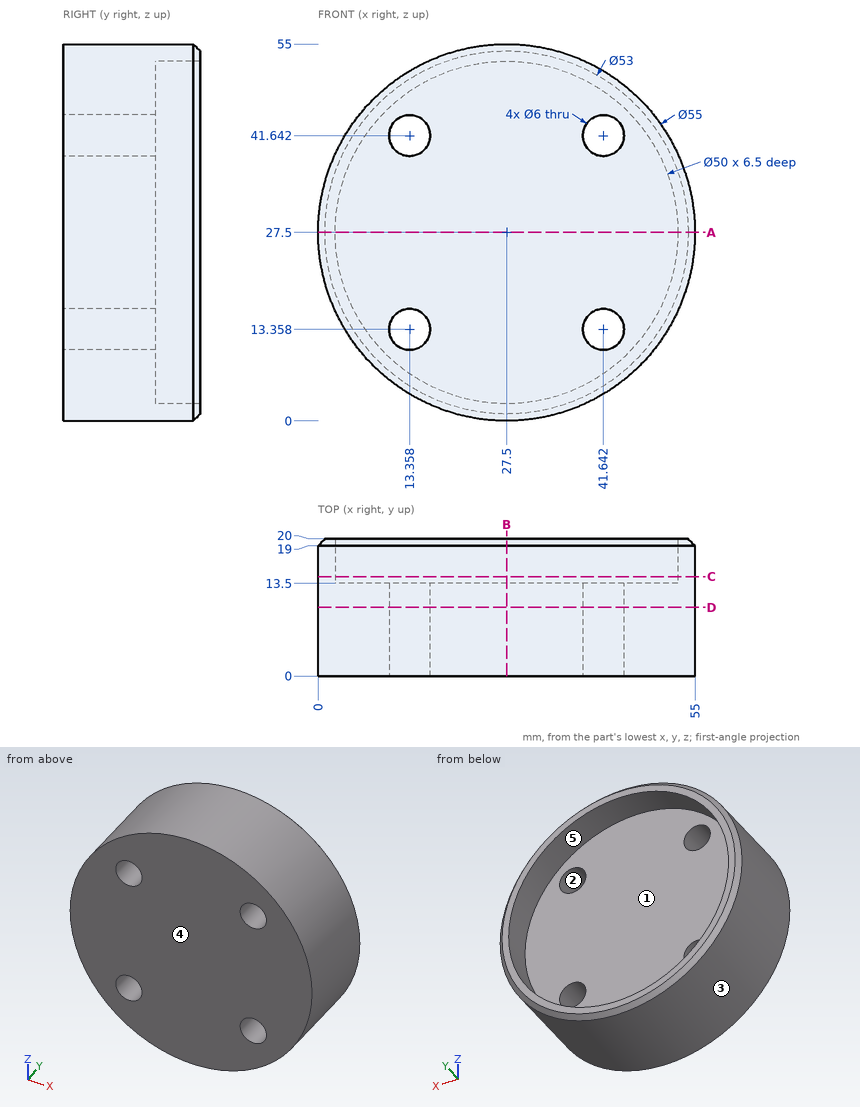
Geometry: see drawing. Coordinates: mm, zero at the bounding-box minimum. A direction names the side the tool comes from. Give positions to 0.01 mm unless a question says otherwise; leave off trailing zeros. Order: outer loops, then holes, each group sorted by start corner. A loop starts at its lowest first (then second) coordinate and runs counter-clockwise, first axis right, second up. Notation, with made-up numbers: (66.5, -32) -> (112.5, -32) arc R19 cw to (112.5, 3) -> close; hole circle Ø11 at (4, 29.25). An arc over 180 degrees is marked (long way). Write each question's results on one line, items separated by ' | '. Start each with the question number.
1) Line query: line 1 (X direction, y = 12, z = 44); line 2 (X direction, y = 11.5, z = 43) (1 decimal); line 3 (Z direction, x = 27.5, y = 16.25). Output: solid intervals per line, ascending. Write a range as from..to.
2) Section D-D (y = 10). Return loops of the section in (x, z), then the cut area to 3 significant figures.
3) Section B-B (x = 27.5). Return loops of the section in (y, z).
4) Section C-C (y = 14.5). Return loops of the section in (x, z), then the cut area to 3 significant figures.
5) Set-up query: the marked faces 1 and 2. Return all of +Z, -Z, +X, -X, +Y, -Y with unobstructed straight access to the full face (end or side cutting, diameter ignored); none if empty.
6) Section A-A (z = 27.5). Return loops of the section in (x, y), then the cut area to 3 significant figures.
7) Draft query along X for the marked faces 3, 4 and 5. Return one class per face: pulls with the +X half, pulls with the -X half, needs draft (parallel to the pull), parting line crosses it, or undercut.
8) First-contact query: pin 1 (2 mm diameter, centred on x = 16.5, z = 42.5, fed in from +Y); pin 2 (8 mm diameter, centred on x = 26, y = 2, fed in from -Z); pin 3 (2 mm diameter, centred on x = 18, y = 4.5, fed in from -Z); pin 4 (3.5 mm diameter, centred on x = 13.36, z = 13.36, fed in from +Y). Flat tips, straight axial feed; report the tip coordinate or a pass-through.
Calculated:
1) line 1: 5.5..11.5, 15.21..39.79, 43.5..49.5 | line 2: 4.8..10.7, 16..39, 44.3..50.2 | line 3: 0..2.5, 52.5..55
2) outline: circle Ø55 at (27.5, 27.5); hole circle Ø6 at (13.36, 13.36); hole circle Ø6 at (13.36, 41.64); hole circle Ø6 at (41.64, 13.36); hole circle Ø6 at (41.64, 41.64) | area: 2,260 mm2
3) outline: (0, 0) -> (19, 0) -> (20, 1) -> (20, 2.5) -> (13.5, 2.5) -> (13.5, 52.5) -> (20, 52.5) -> (20, 54) -> (19, 55) -> (0, 55) -> close
4) outline: circle Ø55 at (27.5, 27.5); hole circle Ø50 at (27.5, 27.5) | area: 412 mm2
5) face 1: +Y | face 2: +Y, -Y
6) outline: (0, 0) -> (55, 0) -> (55, 19) -> (54, 20) -> (52.5, 20) -> (52.5, 13.5) -> (2.5, 13.5) -> (2.5, 20) -> (1, 20) -> (0, 19) -> close | area: 774 mm2
7) face 3: parting line crosses it | face 4: needs draft | face 5: undercut
8) pin 1: y = 13.5 | pin 2: z = 0 | pin 3: z = 1.35 | pin 4: through
